Autodesk Inventor part; units mm, degrees
ref_plane "YZ Plane" through (0, 0, 0) normal (1, 0, 0) x (0, 1, 0)
ref_plane "XZ Plane" through (0, 0, 0) normal (0, 1, 0) x (-1, 0, 0)
sketch "Sketch1" plane through (0, 0, 0) normal (1, 0, 0) x (0, 1, 0)
  line L0 (2.54, 2.54) -> (-48.26, 2.54)
  line L1 (-48.26, 2.54) -> (-48.26, -22.86)
  line L2 (-48.26, -22.86) -> (2.54, -22.86)
  line L3 (2.54, -22.86) -> (2.54, 2.54)
  line L4 (0, 0) -> (-45.72, 0)
  line L5 (-45.72, 0) -> (-45.72, -20.32)
  line L6 (-45.72, -20.32) -> (0, -20.32)
  line L7 (0, -20.32) -> (0, 0)
  dimension "d0" = 50.8
  dimension "d1" = 25.4
  dimension "d5" = 2.54
  dimension "d6" = 2.54
  dimension "d7" = 2.54
  dimension "d8" = 2.54
extrude "Extrusion1" add sketch "Sketch1" along normal blind 444.5
ref_plane "Work Plane1" through (0, -48.26, 1.27) normal (0, 0, 1) x (1, 0, 0)
sketch "Sketch2" plane through (0, -48.26, 1.27) normal (0, 0, 1) x (1, 0, 0)
  line L0 (0, 50.8) -> (444.5, 50.8)
  line L1 (222.25, 50.8) -> (222.25, 0)
  line L2 (0, 0) -> (444.5, 0)
  line L3 (222.25, 25.4) -> (31.75, 25.4)
  line L4 (222.25, 25.4) -> (412.75, 25.4)
  line L5 (222.25, 25.4) -> (222.25, 22.225)
  point P0 (0, 48.26)
  dimension "d11" = 190.5
  dimension "d12" = 190.5
  dimension "d13" = 3.175
  dimension "d14" = 444.5
properties part number "Drive base side"
Verification items for the finished model (mm, model axes). A direction names the side the tool comes from. Round coordinates to 2 decimals unless told otherwise and drop trailing zeros. Loops run counter-clockwise (first coordinate to the right, second up) from the corner with the lowest first, then second, coordinate; pieces in that order, holes last. Notation, with made-up numbers: (-19, 39.5) - (33, 39.5) arc R17 cw to (33, 59.5) - close; hole circle Ø7 at (76.25, 17.5). An arc over 180 degrees is marked (long way). Use one line per item in the form item = value.
1. Scan lines: probe 1 along Y at (x, z) = (160, -9.25); probe 2 along Z at (x, y) = (304.5, -11). Record each from-to range of solid material in increasing order.
A:
probe_1 = -48.26 to -45.72, 0 to 2.54
probe_2 = -22.86 to -20.32, 0 to 2.54
2. Section check A-A on z = -5.5. Record the cut outline in (x, y), and give its area (3 significant figures).
A:
outline = (0, -48.26) - (444.5, -48.26) - (444.5, -45.72) - (0, -45.72) - close; (0, 0) - (444.5, 0) - (444.5, 2.54) - (0, 2.54) - close
area = 2,260 mm²
3. Section check C-C on x = 205.5. Record the cut outline in (y, z), and give its area (3 significant figures).
A:
outline = (-48.26, -22.86) - (2.54, -22.86) - (2.54, 2.54) - (-48.26, 2.54) - close; hole (-45.72, -20.32) - (0, -20.32) - (0, 0) - (-45.72, 0) - close
area = 361 mm²
4. Draft check along Y on faces 1 (the flat face through (219, -45.72, -10)), 2 (the flat face through (0, -23, 0.2)), 3 (the flat face through (219, 2.54, -10)), 4 (the flat face through (219, -23, 0)). Enter one of: pulls with the +Y half, pulls with the -Y half, needs draft (parallel to the pull), parting line crosses it, or undercut.
A:
face_1 = undercut
face_2 = needs draft
face_3 = pulls with the +Y half
face_4 = undercut
5. Section check B-B on y = -12.5. Record the cut outline in (x, z), and give its area (3 significant figures).
A:
outline = (0, -22.86) - (444.5, -22.86) - (444.5, -20.32) - (0, -20.32) - close; (0, 0) - (444.5, 0) - (444.5, 2.54) - (0, 2.54) - close
area = 2,260 mm²
6. Access from +Z, -Z, +X, -X, +Y, -Y to the whole of each face (thin tool, end or side, straight path). Record for faces 5 (the flat face through (219, 0, -10)), 6 (the flat face through (219, -48.26, -10)).
A:
face_5 = +X, -X
face_6 = +Z, -Z, +X, -X, -Y
